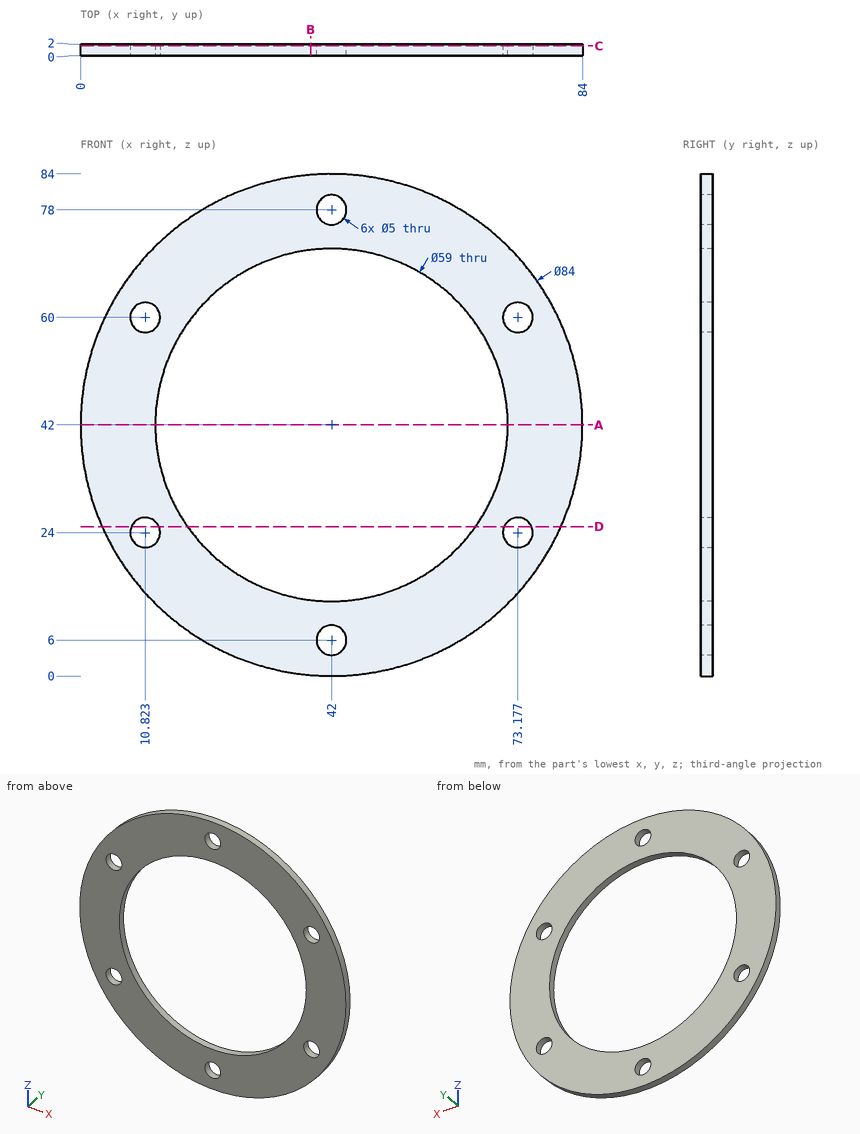
Answer from the drawing. Dimensions are ordinates in mm from the lowest x, y and z of the part. Give positions to 0.01 mm unless a question says otherwise; leave off trailing zeros. Write each loop counter-clockwise with the first axis right and the second up, starting at its lowest first coordinate (ties: lowest second). Pieces come first, ordered by that corner, then holes. Notation, with made-up numbers: (19, 44.5) -> (26, 44.5) arc R31 ccw to (26, 71.5) -> close; hole circle Ø4 at (-26, -22.5). An arc over 180 degrees is marked (long way). One line per question, with ' | ' between items. Start each with the question number.
1. Find the intervals of material crossed by probe 1 along Z at (x, y) = (41.5, 0.7); probe 2 along Z at (x, y) = (10.5, 1.6); probe 3 along X at (y, z) = (1.5, 26), in increasing order.
2. Section D-D (z = 25) is taken. Determine the outline of the cut face in (x, y).
3. Given pin 1 Ø6 at (x, z) = (10.82, 24) entering from +Y, flat-ended and moving along its own axis, determine where the tip first touches the part or whether it passes through.
4. Section A-A (z = 42) is taken. Determine the outline of the cut face in (x, y), plus the area to 3 significant figures.
5. Section C-C (y = 1.7) is taken. Determine the outline of the cut face in (x, z) (3 decimals), plus the area to 3 significant figures.
6. Section B-B (x = 38.5) is taken. Determine the outline of the cut face in (y, z).
Response values:
1) probe 1: 0 to 3.55, 8.45 to 12.5, 71.5 to 75.55, 80.45 to 84 | probe 2: 14.22 to 21.52, 26.48 to 57.52, 62.48 to 69.78 | probe 3: 3.17 to 9.32, 12.32 to 17.22, 66.78 to 71.68, 74.68 to 80.83
2) outline: (3.59, 0) -> (8.53, 0) -> (8.53, 2) -> (3.59, 2) -> close; (13.11, 0) -> (17.89, 0) -> (17.89, 2) -> (13.11, 2) -> close; (66.11, 0) -> (70.89, 0) -> (70.89, 2) -> (66.11, 2) -> close; (75.47, 0) -> (80.41, 0) -> (80.41, 2) -> (75.47, 2) -> close
3) pin 1: y = 2
4) outline: (0, 0) -> (12.5, 0) -> (12.5, 2) -> (0, 2) -> close; (71.5, 0) -> (84, 0) -> (84, 2) -> (71.5, 2) -> close | area: 50.0 mm2
5) outline: circle Ø84 at (42, 42); hole circle Ø5 at (10.823, 24); hole circle Ø5 at (10.823, 60); hole circle Ø59 at (42, 42); hole circle Ø5 at (42, 6); hole circle Ø5 at (42, 78); hole circle Ø5 at (73.177, 24); hole circle Ø5 at (73.177, 60) | area: 2,690 mm2
6) outline: (0, 0.15) -> (2, 0.15) -> (2, 12.71) -> (0, 12.71) -> close; (0, 71.29) -> (2, 71.29) -> (2, 83.85) -> (0, 83.85) -> close
